Build history of the part. All positions in model axes, mm. Face numbers are marked on the shaded views. Round coordinates to 2 decimals unless told otherwise and drop trailing zeros. Loops run counter-clockwise (first coordinate to the right, second up) from the corner with the lowest first, then second, coordinate; pieces in that order, holes last. Notation, with made-up numbers: M 43.5,-36.5 L 51.5,-36.5 A14 cw 51.5,-14.5 Z; hole C 8.5,-34 d4. An arc over 180 degrees is marked long. One line per item, written item: value.
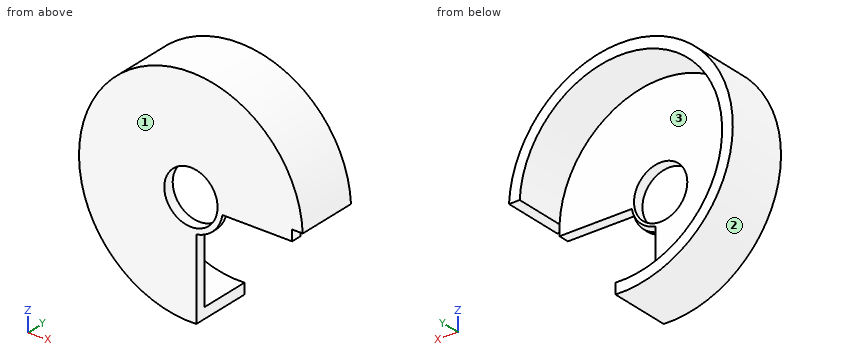
Autodesk Inventor part; units mm, degrees
ref_plane "YZ Plane" through (0, 0, 0) normal (1, 0, 0) x (0, 1, 0)
ref_plane "XZ Plane" through (0, 0, 0) normal (0, 1, 0) x (-1, 0, 0)
ref_plane "XY Plane" through (0, 0, 0) normal (0, 0, 1) x (1, 0, 0)
sketch "Sketch9" plane through (0, 0, 0) normal (0, 1, 0) x (-1, 0, 0)
  arc A0 (-1, -20.9762) -> (-20.9762, 1) centre (0, 0) ccw
  line L0 (21, 0) -> (-21, 0) construction
  line L1 (0, 21) -> (0, -21) construction
  line L2 (21, -1) -> (20.9762, -1)
  line L3 (21, 1) -> (20.9762, 1)
  line L4 (-20.9762, 1) -> (-21, 1)
  line L5 (1, 21) -> (1, 20.9762)
  line L6 (1, -20.9762) -> (1, -21)
  line L7 (-1, 21) -> (-1, 20.9762)
  line L8 (-1, -5.9161) -> (-1, -21)
  line L9 (-5.9161, -1) -> (-18.9762, -1)
  circle A1 centre (0, 0) radius 5
  arc A2 (-5.9161, -1) -> (-1, -5.9161) centre (0, 0) ccw
  line L10 (-20.9762, -1) -> (-18.9762, -1)
  line L11 (-19.9762, -1) -> (-19.9762, 1) construction
  line L12 (-19.9762, 1) -> (-20.9762, 1)
  line L13 (-18.9762, 1) -> (-18.9762, -1)
  line L14 (-18.9762, 1) -> (-19.9762, 1)
  point P0 (-4.899, -1)
  point P1 (-1, -4.899)
  point P2 (-20.9762, -1)
  dimension "d30" = 42
  dimension "d35" = 10
  dimension "d48" = 2
  dimension "d49" = 2
extrude "Extrusion5" add sketch "Sketch9" along normal blind 2
chamfer "Chamfer1" distance 0.5 distance2 1 1 edges at (4.2426, 2, -4.2426) measured on face at (14.1627, 2, 6.4351)
sketch "Sketch10" plane through (0, 2, 0) normal (0, 1, 0) x (1, 0, 0)
  arc A0 (1, 20.9762) -> (20.9762, -1) centre (0, 0) ccw
  arc A1 (1, 18.9737) -> (18.9737, -1) centre (0, 0) ccw
  line L0 (20.058, 1) -> (18.9737, 1)
  line L1 (18.9762, 1) -> (5.4083, 1)
  line L2 (1, 5.4083) -> (1, 20.9762)
  line L3 (1, 18.9737) -> (1, 20.9762)
  line L4 (20.058, 1) -> (20.058, -1) construction
  line L5 (20.058, -1) -> (20.9762, -1)
  line L6 (17.9722, -1) -> (20.9762, -1)
  point P0 (20.9762, 1)
  point P1 (22.9762, 1)
  point P2 (1, 17.9722)
  dimension "d42" = 2
  dimension "d47" = 2
extrude "Extrusion6" add sketch "Sketch10" along normal blind 9.5
properties part number "base layer 1"
Item 1: Pull direction Z, two halves, no side cores. Call the marked faces 1, 2 and 3: pulls with the +Z half, pulls with the -Z half, needs draft (parallel to the pull), parting line crosses it, or undercut.
Check values:
face 1: needs draft
face 2: parting line crosses it
face 3: undercut
Item 2: Slice it at A-A, the plane z = 0. Give the cut face in (x, y).
Check values:
outline: M -21,0 L -5,0 L -5,2 L -19,2 L -19,11.5 L -21,11.5 Z; M 5,0 L 18.98,0 L 18.98,2 L 5,2 Z
Item 3: Slice it at D-D, the plane z = -14. Give the cut face in (x, y).
Check values:
outline: M -15.65,0 L 1,0 L 1,2 L -12.85,2 L -12.85,11.5 L -15.65,11.5 Z
Item 4: Drop flat-ended pins along their axis: P1, Ø3, axis at x = 0, y = 6, coming from the -Z side; P2, Ø8, axis at x = 8, z = 9, coming from the +Y side; P3, Ø1.5, axis at y = 4.5, z = 8, coming from the +X side; P4, Ø1.6, axis at x = 11, y = 0.5, coming from the -Z side. Give the stop position or say it passes through.
Check values:
P1: stops at z = -21
P2: stops at y = 2
P3: stops at x = 19.71
P4: stops at z = -1
Item 5: Wall check: line 1 along Z through (x, y) = (0, 4.5); line 2 along Y through (x, z) = (7.5, 16); line 3 along X through (y, z) = (5.75, 0). Give the ranges that are in metal, low to high.
Check values:
line 1: z = -21 to -19, 19 to 21
line 2: y = 0 to 2
line 3: x = -21 to -19
Item 6: Slice it at C-C, the plane x = -11.5. Give the cut face in (y, z).
Check values:
outline: M 0,-17.57 L 11.5,-17.57 L 11.5,-15.12 L 2,-15.12 L 2,15.12 L 11.5,15.12 L 11.5,17.57 L 0,17.57 Z
Item 7: Slice it at B-B, the plane x = 0. Give the cut face in (y, z).
Check values:
outline: M 0,-21 L 11.5,-21 L 11.5,-19 L 2,-19 L 2,-5 L 0,-5 Z; M 0,5 L 2,5 L 2,19 L 11.5,19 L 11.5,21 L 0,21 Z
